```python
from build123d import *

# Parameters (mm, degrees)
F0_R     = 2.5
F1_DEPTH = 1


with BuildPart() as f1:
    # F0 (on Top) → F1 (new body)
    with BuildSketch(Plane.XY):
        with BuildLine():
            Line((-24.598089, 25.583514), (-49.598089, 50.583514))
            ThreePointArc((-49.598089, 50.583514), (-67.275759, 50.583514), (-67.275759, 32.905845))
            Line((-67.275759, 32.905845), (-42.275759, 7.905845))
            ThreePointArc((-42.275759, 7.905845), (-35.577566, -9.360294), (-43.809394, -25.95012))
            Line((-43.809394, -25.95012), (-67.275759, -49.416486))
            ThreePointArc((-67.275759, -49.416486), (-67.275759, -67.094155), (-49.598089, -67.094155))
            Line((-49.598089, -67.094155), (-24.598089, -42.094155))
            ThreePointArc((-24.598089, -42.094155), (-8.436924, -35.399981), (7.724241, -42.094155))
            Line((7.724241, -42.094155), (32.724241, -67.094155))
            ThreePointArc((32.724241, -67.094155), (50.401911, -67.094155), (50.401911, -49.416486))
            Line((50.401911, -49.416486), (26.404182, -25.418757))
            ThreePointArc((26.404182, -25.418757), (18.705964, -8.972916), (25.401911, 7.905845))
            Line((25.401911, 7.905845), (50.401911, 32.905845))
            ThreePointArc((50.401911, 32.905845), (50.401911, 50.583514), (32.724241, 50.583514))
            Line((32.724241, 50.583514), (7.724241, 25.583514))
            ThreePointArc((7.724241, 25.583514), (-8.436924, 18.889341), (-24.598089, 25.583514))
        make_face()
        with Locations((-58.436924, -58.25532)):
            Circle(F0_R, mode=Mode.SUBTRACT)
        with Locations((41.563076, -58.25532)):
            Circle(F0_R, mode=Mode.SUBTRACT)
        with Locations((-58.436924, 41.74468)):
            Circle(F0_R, mode=Mode.SUBTRACT)
        with Locations((41.563076, 41.74468)):
            Circle(F0_R, mode=Mode.SUBTRACT)
    extrude(amount=F1_DEPTH)


solid = f1.part
```
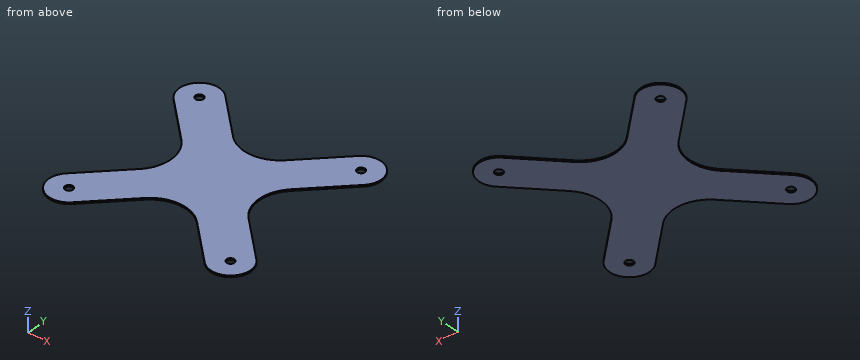
Design review of the part built by this model. Coordinates are the model's own, in mm. Coordinates: 2 decimals unless noted, no trailing zeros. Loops run counter-clockwise (first coordinate to the right, second up) from the corner with the lowest first, then second, coordinate; pieces in that order, holes last. Notation, with made-up numbers: (-28, 48) -> (-19, 48) arc R4 cw to (-19, 52) -> close; hole circle Ø1 at (84.25, 89.5). An arc over 180 degrees is marked (long way). Answer as a JSON object with one key per item and string values.
Q1. Take a section at D-D on y = 3. Give the boundary of the cut face in (x, z), plus the area to 3 significant figures.
Answer block:
{"outline": "(-38.54, 0) -> (21.67, 0) -> (21.67, 1) -> (-38.54, 1) -> close", "area": "60.2 mm^2"}
Q2. Take a section at B-B on x = 29.5. Give the boundary of the cut face in (y, z).
Answer block:
{"outline": "(-63.87, 0) -> (-28.51, 0) -> (-28.51, 1) -> (-63.87, 1) -> close; (12, 0) -> (47.36, 0) -> (47.36, 1) -> (12, 1) -> close"}
Q3. Take a section at C-C on z = 0.4. Give the boundary of the cut face in (x, y).
Answer block:
{"outline": "(-67.28, -49.42) arc R12.5 ccw to (-49.6, -67.09) -> (-24.6, -42.09) arc R22.86 cw to (7.72, -42.09) -> (32.72, -67.09) arc R12.5 ccw to (50.4, -49.42) -> (26.4, -25.42) arc R22.9 cw to (25.4, 7.91) -> (50.4, 32.91) arc R12.5 ccw to (32.72, 50.58) -> (7.72, 25.58) arc R22.86 cw to (-24.6, 25.58) -> (-49.6, 50.58) arc R12.5 ccw to (-67.28, 32.91) -> (-42.28, 7.91) arc R22.95 cw to (-43.81, -25.95) -> close; hole circle Ø5 at (-58.44, -58.26); hole circle Ø5 at (-58.44, 41.74); hole circle Ø5 at (41.56, -58.26); hole circle Ø5 at (41.56, 41.74)"}
Q4. Take a section at A-A on y = 47. Give the boundary of the cut face in (x, z), plus the area to 3 significant figures.
Answer block:
{"outline": "(-69.78, 0) -> (-46.01, 0) -> (-46.01, 1) -> (-69.78, 1) -> close; (29.14, 0) -> (52.9, 0) -> (52.9, 1) -> (29.14, 1) -> close", "area": "47.5 mm^2"}
Q5. To check wall thickness, follow L1, parallel to Y at x = -53, z = 0.8; L2, parallel to X at y = -66, z = 0.6; L3, parallel to X at y = 31, z = 0.2. State the ranges of each line that lie inside material, in increasing order.
Answer block:
{"L1": "y = -69.51 to -35.14, 18.63 to 53", "L2": "x = -68.25 to -48.5, 31.63 to 51.37", "L3": "x = -65.37 to -30.01, 13.14 to 48.5"}
